Autodesk Inventor part; units mm, degrees
ref_plane "YZ Plane" through (0, 0, 0) normal (1, 0, 0) x (0, 1, 0)
ref_plane "XZ Plane" through (0, 0, 0) normal (0, 1, 0) x (-1, 0, 0)
ref_plane "XY Plane" through (0, 0, 0) normal (0, 0, 1) x (1, 0, 0)
sketch "Boceto1" plane through (0, 0, 0) normal (0, 0, 1) x (1, 0, 0)
  line L0 (0, 0) -> (80, 0)
  line L1 (80, 0) -> (80, 230)
  line L2 (80, 230) -> (0, 230)
  line L3 (0, 230) -> (0, 0)
  dimension "d0" = 80
  dimension "d1" = 230
extrude "Extrusión1" add sketch "Boceto1" along normal blind 3
sketch "Boceto2" plane through (0, 0, 3) normal (0, 0, 1) x (1, 0, 0)
  line L0 (0, 0) -> (80, 0) construction
  line L1 (80, 0) -> (80, 230) construction
  line L2 (80, 230) -> (0, 230) construction
  line L3 (0, 230) -> (0, 0) construction
  line L4 (3, 0) -> (0, 0)
  line L5 (0, 0) -> (0, 50)
  line L6 (0, 50) -> (3, 50)
  line L7 (3, 50) -> (3, 0)
  line L8 (0, 230) -> (17.5445, 230)
  line L9 (77, 100) -> (80, 100)
  line L10 (80, 100) -> (80, 50)
  line L11 (80, 50) -> (77, 50)
  line L12 (77, 50) -> (77, 100)
  line L13 (80, 0) -> (80, 230) construction
  line L14 (0, 150) -> (3, 150)
  line L15 (3, 150) -> (3, 100)
  line L16 (3, 100) -> (0, 100)
  line L17 (0, 100) -> (0, 150)
  line L18 (0, 230) -> (0, 0) construction
  point P0 (80, 115)
  dimension "d4" = 3
  dimension "d5" = 50
  dimension "d8" = 50
  dimension "d9" = 3
  dimension "d16" = 50
  dimension "d17" = 3
  dimension "d18" = 50
  dimension "d19" = 50
extrude "Extrusión2" cut sketch "Boceto2" against normal blind 3
sketch "Boceto3" plane through (0, 0, 3) normal (0, 0, 1) x (1, 0, 0)
  line L0 (3, 50) -> (3, 0) construction
  line L1 (3, 0) -> (80, 0) construction
  line L2 (80, 0) -> (80, 50) construction
  line L3 (80, 50) -> (77, 50) construction
  line L4 (77, 50) -> (77, 100) construction
  line L5 (77, 100) -> (80, 100) construction
  line L6 (80, 100) -> (80, 230) construction
  line L7 (80, 230) -> (0, 230) construction
  line L8 (0, 230) -> (0, 150) construction
  line L9 (0, 50) -> (3, 50) construction
  line L10 (40, 70) -> (43, 70)
  line L11 (43, 70) -> (43, 0)
  line L12 (43, 0) -> (40, 0)
  line L13 (40, 0) -> (40, 70)
  line L14 (3, 0) -> (80, 0) construction
  line L15 (0, 150) -> (3, 150)
  line L16 (3, 150) -> (3, 100)
  line L17 (3, 100) -> (0, 100)
  line L18 (0, 100) -> (0, 50)
  point P0 (0, 0)
  point P1 (41.5, 0)
  point P2 (41.5, 0)
  dimension "d12" = 3
  dimension "d13" = 70
extrude "Extrusión3" cut sketch "Boceto3" against normal blind 10
sketch "Boceto4" plane through (0, 0, 3) normal (0, 0, 1) x (1, 0, 0)
  line L0 (43, 70) -> (43, 0) construction
  line L1 (43, 0) -> (80, 0) construction
  line L2 (80, 0) -> (80, 50) construction
  line L3 (80, 50) -> (77, 50) construction
  line L4 (77, 50) -> (77, 100) construction
  line L5 (77, 100) -> (80, 100) construction
  line L6 (80, 100) -> (80, 230) construction
  line L7 (80, 230) -> (0, 230) construction
  line L8 (0, 230) -> (0, 150) construction
  line L9 (0, 150) -> (3, 150) construction
  line L10 (3, 150) -> (3, 100) construction
  line L11 (3, 100) -> (0, 100) construction
  line L12 (0, 100) -> (0, 50) construction
  line L13 (0, 50) -> (3, 50) construction
  line L14 (3, 50) -> (3, 0) construction
  line L15 (3, 0) -> (40, 0) construction
  line L16 (40, 0) -> (40, 70) construction
  line L17 (40, 70) -> (43, 70) construction
  point P0 (0, 0)
  point P1 (25, 200)
  point P2 (55, 200)
  dimension "d20" = 30
  dimension "d21" = 30
  dimension "d23" = 25
  dimension "d24" = 30
hole "Agujero1" at (25, 200, 3) at (55, 200, 3) direction (0, 0, -1) diameter 3.3 end through all both
sketch "Boceto5" plane through (0, 0, 3) normal (0, 0, 1) x (1, 0, 0)
  circle A0 centre (25, 200) radius 1.65 construction
  circle A1 centre (55, 200) radius 1.65 construction
  line L0 (43, 70) -> (43, 0) construction
  line L1 (43, 0) -> (80, 0) construction
  line L2 (80, 0) -> (80, 50) construction
  line L3 (80, 50) -> (77, 50) construction
  line L4 (77, 50) -> (77, 100) construction
  line L5 (77, 100) -> (80, 100) construction
  line L6 (80, 100) -> (80, 230) construction
  line L7 (80, 230) -> (0, 230) construction
  line L8 (0, 230) -> (0, 150) construction
  line L9 (0, 150) -> (3, 150) construction
  line L10 (3, 150) -> (3, 100) construction
  line L11 (3, 100) -> (0, 100) construction
  line L12 (0, 100) -> (0, 50) construction
  line L13 (0, 50) -> (3, 50) construction
  line L14 (3, 50) -> (3, 0) construction
  line L15 (3, 0) -> (40, 0) construction
  line L16 (40, 0) -> (40, 70) construction
  line L17 (40, 70) -> (43, 70) construction
  line L18 (14, 3) -> (29, 3)
  line L19 (29, 3) -> (29, 0)
  line L20 (29, 0) -> (14, 0)
  line L21 (14, 0) -> (14, 3)
  line L22 (54, 3) -> (69, 3)
  line L23 (69, 3) -> (69, 0)
  line L24 (69, 0) -> (54, 0)
  line L25 (54, 0) -> (54, 3)
  line L26 (3, 0) -> (40, 0) construction
  line L27 (43, 0) -> (80, 0) construction
  point P0 (0, 0)
  point P1 (21.5, 0)
  point P2 (21.5, 0)
  point P3 (61.5, 0)
  point P4 (61.5, 0)
  dimension "d32" = 3
  dimension "d33" = 3
  dimension "d35" = 15
  dimension "d36" = 15
extrude "Extrusión4" cut sketch "Boceto5" against normal blind 10
equation "\"d8\" = d7"
equation "\"d9\" = d4"
equation "\"d7\" = d5"
properties part number "Pared Garita3"
Input: part model. Units: mm. Frame: model coordinates. Coordinates: 2 decimals unless noted, no trailing zeros. Write each loop counter-clockwise with the first axis right and the second up, starting at its lowest first coordinate (ties: lowest second). Pieces come first, ordered by that corner, then holes.
1) Pin query (flat end, axial travel): pin 1 Ø1.5 at (x, z) = (57, 1) entering from -Y; pin 2 Ø1.5 at (y, z) = (1, 1.5) entering from -X; pin 3 Ø0.9 at (x, z) = (41.5, 2) entering from -Y. Return the tip coordinate at first contact, or that it passes through.
2) Section A-A on z = 0.7. Output: boundary loops of the cut face in (x, y), and give its area (3 significant figures).
3) Material intervals for line 1 along X through (y, z) = (200, 1.05); line 2 along X through (y, z) = (65, 2.15); line 3 along Y through (x, z) = (25, 1.1), sorted ascending.
Check result:
1. pin 1: stops at y = 3
1. pin 2: stops at x = 3
1. pin 3: stops at y = 70
2. outline: (0, 50) - (3, 50) - (3, 0) - (14, 0) - (14, 3) - (29, 3) - (29, 0) - (40, 0) - (40, 70) - (43, 70) - (43, 0) - (54, 0) - (54, 3) - (69, 3) - (69, 0) - (80, 0) - (80, 50) - (77, 50) - (77, 100) - (80, 100) - (80, 230) - (0, 230) - (0, 150) - (3, 150) - (3, 100) - (0, 100) - close; hole circle Ø3.3 at (25, 200); hole circle Ø3.3 at (55, 200)
2. area: 17,600 mm2
3. line 1: x = 0 to 23.35, 26.65 to 53.35, 56.65 to 80
3. line 2: x = 0 to 40, 43 to 77
3. line 3: y = 3 to 198.35, 201.65 to 230
